Here's how the part is built. I have some questions about the finished solid (model axes, mm). A direction names the side the tool comes from. Coordinates: 2 decimals unless noted, no trailing zeros. Order: outer loops, then holes, each group sorted by start corner. A loop starts at its lowest first (then second) coordinate and runs counter-clockwise, first axis right, second up. Notation, with made-up numbers: (66.5, 83) - (73.5, 83) arc R18 cw to (73.5, 96) - close; hole circle Ø10 at (35, 52.5). An arc over 180 degrees is marked (long way). Answer in a Markdown table with one row per item. Add a question column.
Item 1: I want a section at C-C (y = -244.5). Please give me the cut outline in (x, z).
Item 2: I want a section at B-B (x = -107). Please give me the cut outline in (y, z).
Item 3: Thinking about a two-plate mould opening in Y: for faces 1 (the flat face through (-145, -221, 2)), 2 (the flat face through (-143, -135.937, 2)), 3 (the flat face through (-143, -175.937, 2)), which applies, +Y half, -Y half, draft (parallel to the pull), parting line (faces both ways), or undercut?
Item 4: Will these pins go through, and if not, where does the flat tip stop? pin 1 Ø2 at (y, z) = (-188, 1.5) entering from -X; pin 2 Ø1.2 at (y, z) = (-255.5, 1.5) entering from -X; pin 3 Ø1.2 at (y, z) = (-256, 2) entering from +X; pin 4 Ø3 at (x, y) = (-128.5, -192.5) entering from -Z.
Item 5: If I drill on line 1 along Y through (x, z) = (-128, 2.4); line 2 along Y through (x, z) = (-100, 1.9); line 3 along X through (y, z) = (-244, 3.85), over which ranges is the centre line in solid material (lowest first)? Write a range as from..to.
Item 6: I want a section at A-A (z = 3.1). Please give me the cut outline in (x, y), plus the area to 3 significant figures.
Item 7: On a 3-axis mill with a long thin cutter (end or side, diameter ignored), from which of +Z, -Z, +X, -X, +Y, -Y can I reach the whole of each face in a straight line? I mean faces 4 (the flat face through (-143, -200.839, 2)), 5 (the flat face through (-99, -240.839, 2)), 6 (the flat face through (-126, -256, 2)). Say none if no direction works.
Autodesk Inventor part; units mm, degrees
ref_plane "Work Plane1" through (-101, -191.2, 4) normal (0, 1, 0) x (1, 0, 0)
ref_plane "YZ Plane" through (0, 0, 0) normal (1, 0, 0) x (0, 1, 0)
ref_plane "XZ Plane" through (0, 0, 0) normal (0, 1, 0) x (-1, 0, 0)
sketch "Sketch1" plane through (0, 0, 0) normal (0, 0, 1) x (1, 0, 0)
  line L0 (-101, -200.839) -> (-97, -200.839)
  line L1 (-97, -200.839) -> (-97, -240.839)
  line L2 (-97, -240.839) -> (-101, -240.839)
  line L3 (-101, -240.839) -> (-101, -258.2)
  line L4 (-101, -128.2) -> (-101, -135.9372)
  line L5 (-101, -135.9372) -> (-97, -135.9372)
  line L6 (-97, -135.9372) -> (-97, -175.9372)
  line L7 (-97, -175.9372) -> (-101, -175.9372)
  line L8 (-101, -175.9372) -> (-101, -200.839)
  line L9 (-101, -258.2) -> (-101, -254.2)
  line L10 (-101, -254.2) -> (-141, -254.2)
  line L11 (-101, -128.2) -> (-141, -128.2)
  line L12 (-121, -128.2) -> (-121, -103.1789)
  line L13 (-145, -200.839) -> (-145, -240.839)
  line L14 (-145, -240.839) -> (-141, -240.839)
  line L15 (-141, -200.839) -> (-145, -200.839)
  line L16 (-145, -175.9372) -> (-141, -175.9372)
  line L17 (-145, -135.9372) -> (-145, -175.9372)
  line L18 (-141, -135.9372) -> (-145, -135.9372)
  line L19 (-141, -135.9372) -> (-141, -128.2)
  line L20 (-141, -254.2) -> (-141, -240.839)
  line L21 (-141, -200.839) -> (-141, -175.9372)
  point P0 (0, 0)
  dimension "d0" = 4
  dimension "d1" = 40
  dimension "d2" = 40
  dimension "d3" = 40
extrude "Extrusion1" add sketch "Sketch1" along normal blind 4
sketch "Sketch2" plane through (0, 0, 4) normal (0, 0, 1) x (1, 0, 0)
  line L0 (-97, -200.839) -> (-101, -200.839)
  line L1 (-101, -200.839) -> (-101, -175.9372)
  line L2 (-101, -175.9372) -> (-97, -175.9372)
  line L3 (-97, -175.9372) -> (-97, -135.9372)
  line L4 (-97, -135.9372) -> (-101, -135.9372)
  line L5 (-101, -135.9372) -> (-101, -128.2)
  line L6 (-101, -128.2) -> (-141, -128.2)
  line L7 (-141, -128.2) -> (-141, -135.9372)
  line L8 (-141, -135.9372) -> (-145, -135.9372)
  line L9 (-145, -135.9372) -> (-145, -175.9372)
  line L10 (-145, -175.9372) -> (-141, -175.9372)
  line L11 (-141, -175.9372) -> (-141, -200.839)
  line L12 (-141, -200.839) -> (-145, -200.839)
  line L13 (-145, -200.839) -> (-145, -240.839)
  line L14 (-145, -240.839) -> (-141, -240.839)
  line L15 (-141, -240.839) -> (-141, -254.2)
  line L16 (-141, -254.2) -> (-101, -254.2)
  line L17 (-101, -254.2) -> (-101, -240.839)
  line L18 (-101, -240.839) -> (-97, -240.839)
  line L19 (-97, -240.839) -> (-97, -200.839)
  line L20 (-126, -128.2) -> (-116, -128.2)
  line L21 (-116, -128.2) -> (-116, -124.2)
  line L22 (-116, -124.2) -> (-126, -124.2)
  line L23 (-126, -124.2) -> (-126, -128.2)
  point P0 (0, 0)
  point P1 (-121, -128.2)
  dimension "d6" = 10
  dimension "d7" = 4
extrude "Extrusion2" add sketch "Sketch2" against normal blind 4 contours L6 L23 L22 L21
ref_plane "Work Plane1" through (-101, -191.2, 4) normal (0, 1, 0) x (1, 0, 0)
mirror "Mirror1" about plane through (-101, -191.2, 4) normal (0, 1, 0) of "Extrusion2"
properties part number "F7"
Values follow:
| question | item | result |
|---|---|---|
| 1 | outline | (-141, 0) - (-101, 0) - (-101, 4) - (-141, 4) - close |
| 2 | outline | (-254.2, 0) - (-128.2, 0) - (-128.2, 4) - (-254.2, 4) - close |
| 3 | face 1 | draft |
| 3 | face 2 | +Y half |
| 3 | face 3 | undercut |
| 4 | pin 1 | stops at x = -141 |
| 4 | pin 2 | stops at x = -126 |
| 4 | pin 3 | stops at x = -116 |
| 4 | pin 4 | stops at z = 0 |
| 5 | line 1 | y = -254.2..-128.2 |
| 5 | line 2 | y = -240.84..-200.84, -175.94..-135.94 |
| 5 | line 3 | x = -141..-101 |
| 6 | outline | (-145, -240.84) - (-141, -240.84) - (-141, -254.2) - (-126, -254.2) - (-126, -258.2) - (-116, -258.2) - (-116, -254.2) - (-101, -254.2) - (-101, -240.84) - (-97, -240.84) - (-97, -200.84) - (-101, -200.84) - (-101, -175.94) - (-97, -175.94) - (-97, -135.94) - (-101, -135.94) - (-101, -128.2) - (-116, -128.2) - (-116, -124.2) - (-126, -124.2) - (-126, -128.2) - (-141, -128.2) - (-141, -135.94) - (-145, -135.94) - (-145, -175.94) - (-141, -175.94) - (-141, -200.84) - (-145, -200.84) - close |
| 6 | area | 5,760 mm^2 |
| 7 | face 4 | +Z, -Z, -X |
| 7 | face 5 | +Z, -Z, +X, -Y |
| 7 | face 6 | +Z, -Z, -X, -Y |
